Source: three-view drawing plus pictorial views. Frame: mm from the lowest corner of the part. A direction names the side the tool comes from. Give positions to 0.01 mm unless a question says otherwise; leave off trailing zeros. Loops run counter-clockwise (first coordinate to the right, second up) from the corner with the lowest first, then second, coordinate; pieces in that order, holes last.
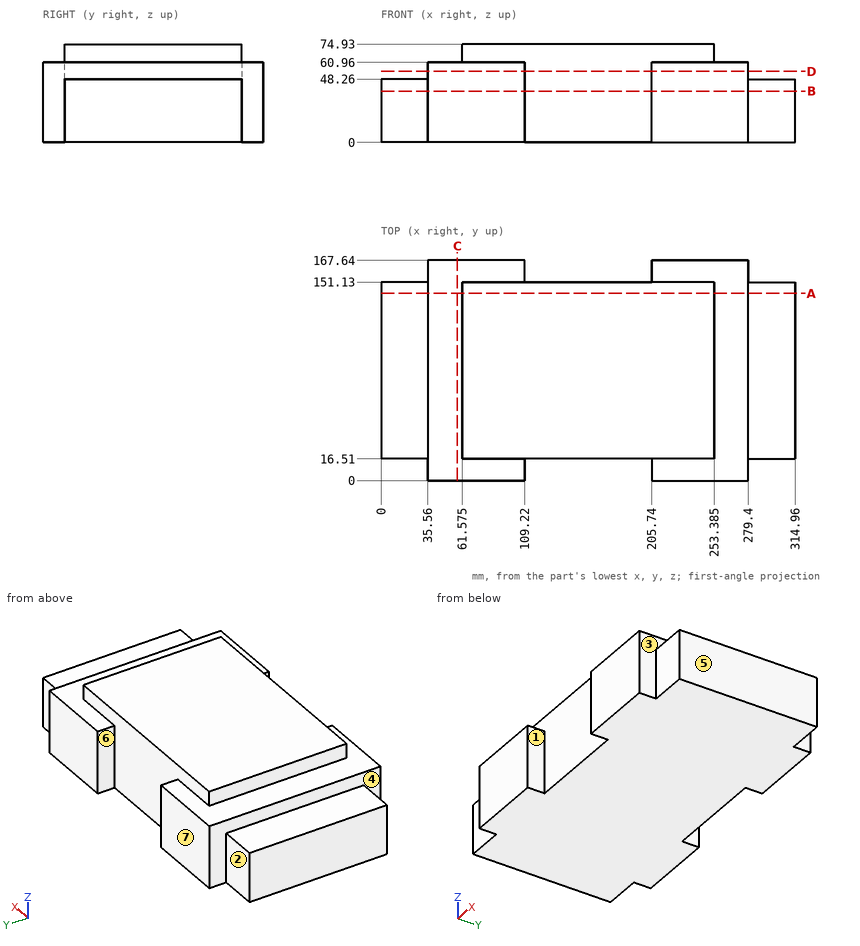
Q1. Material intervals for probe 1 along X at (y, z) = (151.5, 43); probe 2 along X at (y, z) = (54, 71.5) (1 decimal); probe 3 along X at (y, z) = (127.5, 56.5), sorted ascending.
Q2. Pin query (flat end, axial travel): pin 1 Ø18 at (x, y) = (26, 69.5) entering from +Z; pin 2 Ø10.5 at (x, z) = (23, 26.5) entering from -Y; pin 3 Ø2 at (y, z) = (44, 53) entering from -X. Return the tip coordinate at first contact, or that it passes through.
Q3. Section query A-A, the plane y = 142.5. Return loops of the section in (x, z) (1 decimal).
Q4. Section query B-B, the plane z = 39. Return loops of the section in (x, y), and give its area (3 significant figures).
Q5. Reachability of the marked faces 1, 2 and 3 from +Z, -Z, +X, -X, +Y, -Y: full face, straight path, thin tool, end or side. Return the list, or none.
Q6. Mould query, pull axis X, two halves, no side actions, for the marked faces 4, 5, 6 and 7. Classes: +X half, -X half, draft (parallel to the pull), parting line (faces both ways), or undercut.
Q7. Section query C-C, the plane x = 58. Return loops of the section in (y, z).
Q8. Section query D-D, the plane z = 54. Return loops of the section in (x, y), and give its area (3 significant figures).
Resolved:
1. probe 1: x = 35.56 to 109.22, 205.74 to 279.4
1. probe 2: x = 61.6 to 253.4
1. probe 3: x = 35.56 to 279.4
2. pin 1: stops at z = 48.26
2. pin 2: stops at y = 16.51
2. pin 3: stops at x = 35.56
3. outline: (0, 0) - (315, 0) - (315, 48.3) - (279.4, 48.3) - (279.4, 61) - (253.4, 61) - (253.4, 74.9) - (61.6, 74.9) - (61.6, 61) - (35.6, 61) - (35.6, 48.3) - (0, 48.3) - close
4. outline: (0, 16.51) - (35.56, 16.51) - (35.56, 0) - (109.22, 0) - (109.22, 16.51) - (205.74, 16.51) - (205.74, 0) - (279.4, 0) - (279.4, 16.51) - (314.96, 16.51) - (314.96, 151.13) - (279.4, 151.13) - (279.4, 167.64) - (205.74, 167.64) - (205.74, 151.13) - (109.22, 151.13) - (109.22, 167.64) - (35.56, 167.64) - (35.56, 151.13) - (0, 151.13) - close
4. area: 47,300 mm2
5. face 1: +Z, -Z, -Y
5. face 2: +Z, -Z, -X, +Y
5. face 3: +Z, +X
6. face 4: -X half
6. face 5: +X half
6. face 6: undercut
6. face 7: draft
7. outline: (0, 0) - (167.64, 0) - (167.64, 60.96) - (0, 60.96) - close
8. outline: (35.56, 0) - (109.22, 0) - (109.22, 16.51) - (205.74, 16.51) - (205.74, 0) - (279.4, 0) - (279.4, 167.64) - (205.74, 167.64) - (205.74, 151.13) - (109.22, 151.13) - (109.22, 167.64) - (35.56, 167.64) - close
8. area: 37,700 mm2
